For this review, use the dimensioned drawing (mm, ordinates from the lowest corner) and the shaded views. Round coordinates to 2 decimals unless told otherwise and drop trailing zeros. Order: outer loops, then holes, each group sorted by start corner. A loop starts at its lowest first (then second) coordinate and runs counter-clockwise, first axis right, second up. Notation, with made-up numbers: M 76.25,-11 L 83.25,-11 A21 cw 83.25,21 Z; hole C -33.75,-11.75 d10. An arc over 180 degrees is marked long. One line per item, written item: value. Start each with the question number.
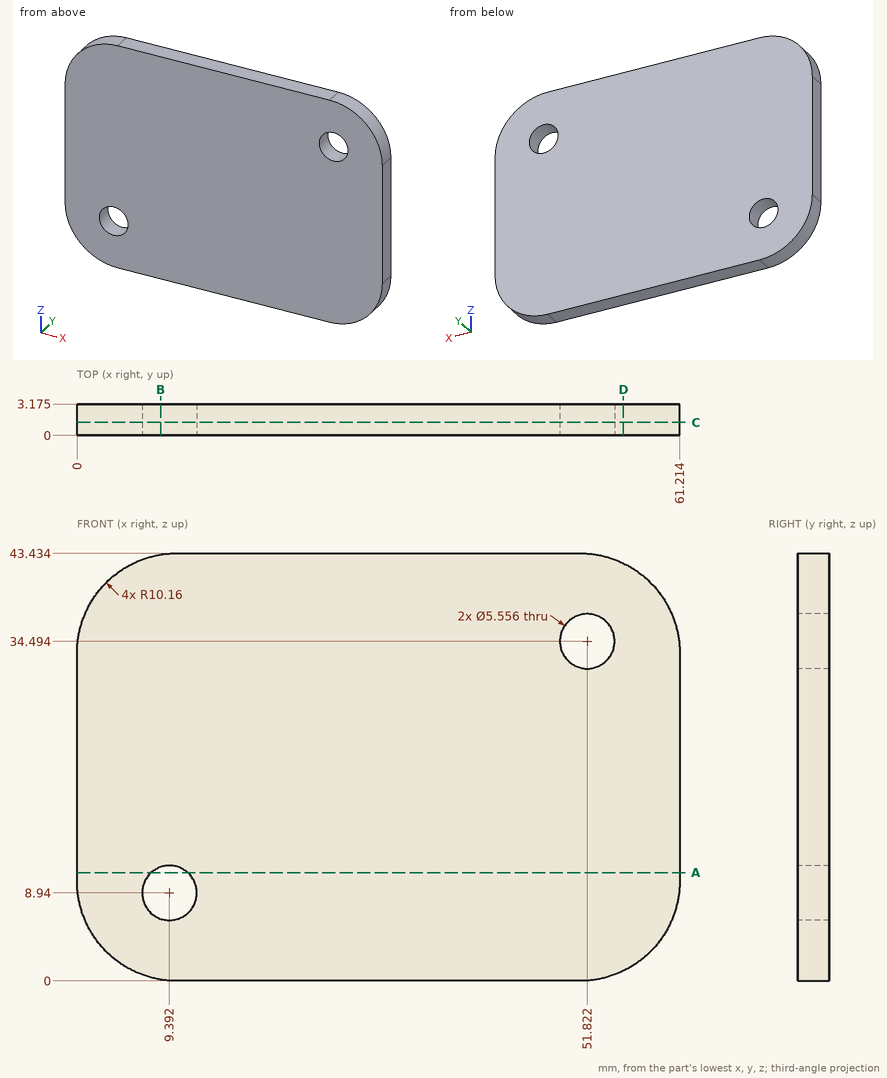
Item 1: Consider section C-C, the plane y = 1.3. Give the boundary of the cut face in (x, z) (1 decimal), then the cut area to 3 significant figures.
Item 2: Consider section D-D, the plane x = 55.5. Give the boundary of the cut face in (y, z) (1 decimal).
Item 3: Consider section A-A, the plane z = 11. Give the boundary of the cut face in (x, y) (1 decimal).
Item 4: Wall thickness on L1, parallel to X at y = 2.15, z = 34 (1 decimal); L2, parallel to X at y = 0.7, z = 35 (1 decimal); L3, parallel to X at y = 1, z = 42 (1 decimal): over which ranges is each line inside the solid? List them lowest first.
Item 5: Consider section B-B, the plane x = 8.5. Give the boundary of the cut face in (y, z) (1 decimal), then the cut area to 3 significant figures.
Computed:
1. outline: M 0,10.2 A10.2 ccw 10.2,0 L 51.1,0 A10.2 ccw 61.2,10.2 L 61.2,33.3 A10.2 ccw 51.1,43.4 L 10.2,43.4 A10.2 ccw 0,33.3 Z; hole C 9.4,8.9 d5.6; hole C 51.8,34.5 d5.6
1. area: 2,520 mm^2
2. outline: M 0,1 L 3.2,1 L 3.2,42.4 L 0,42.4 Z
3. outline: M 0,0 L 7.5,0 L 7.5,3.2 L 0,3.2 Z; M 11.3,0 L 61.2,0 L 61.2,3.2 L 11.3,3.2 Z
4. L1: x = 0 to 49.1, 54.6 to 61.2
4. L2: x = 0.1 to 49.1, 54.6 to 61.1
4. L3: x = 5 to 56.3
5. outline: M 0,0.1 L 3.2,0.1 L 3.2,6.3 L 0,6.3 Z; M 0,11.6 L 3.2,11.6 L 3.2,43.3 L 0,43.3 Z
5. area: 120 mm^2
